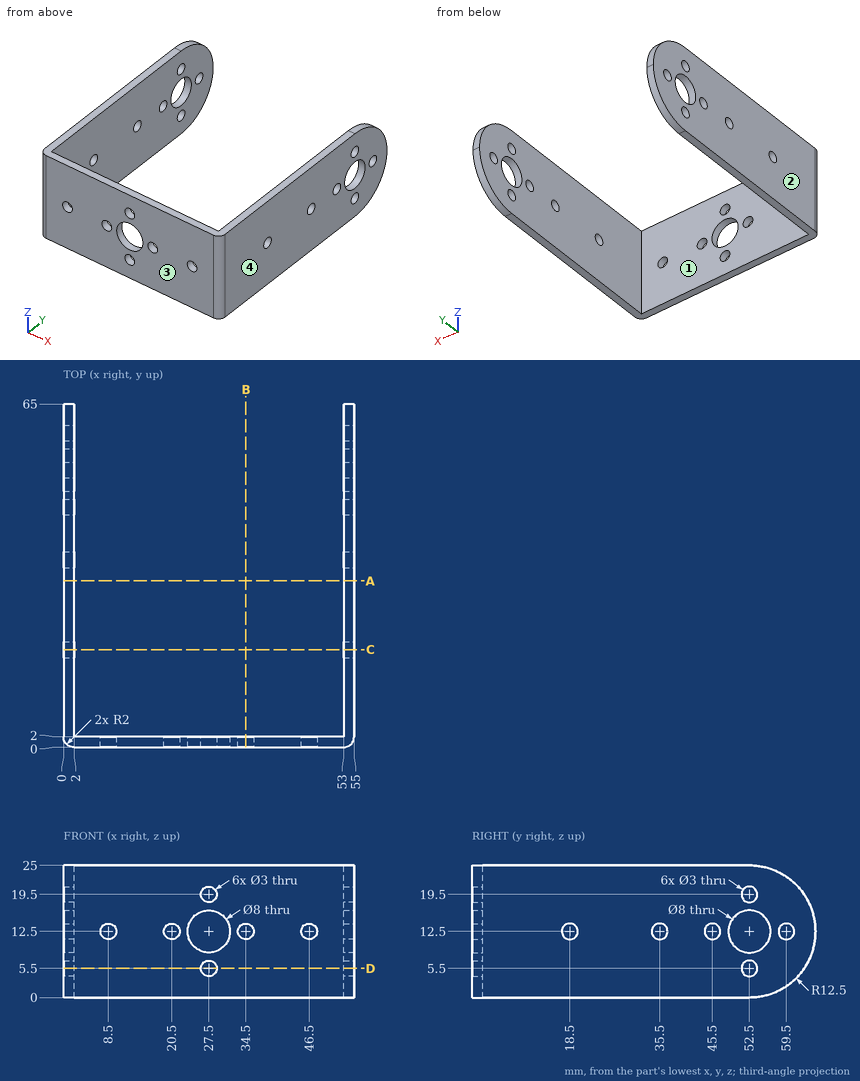
Could you check a few things on this drawing? It's one solid part, dimensions in mm from its lowest x, y, z. Give positions to 0.01 mm unless a question says otherwise; leave off trailing zeros. Write each loop counter-clockwise with the first axis right and the second up, starting at its lowest first coordinate (ties: lowest second). Pieces come first, ordered by that corner, then holes. Notation, with made-up numbers: (-26.75, 20) -> (1.25, 20) arc R13 ccw to (1.25, 37) -> close; hole circle Ø9 at (49, 37). An arc over 180 degrees is marked (long way). Write item = value, one per line.
(1) Suppose I cut it at B-B on x = 34.5. Write out the boundary of the cut face in (y, z).
Worked out:
outline = (0, 0) -> (2, 0) -> (2, 11) -> (0, 11) -> close; (0, 14) -> (2, 14) -> (2, 25) -> (0, 25) -> close
(2) I need wall thicknesses on probe 1 along Z at (x, y) = (27.5, 1.05); probe 2 along X at (y, z) = (59, 8); probe 3 along Y at (x, z) = (48, 6.25). Which ranges of each line are inside material? Lowest first, please. Write a range as from..to.
Worked out:
probe_1 = 0..4, 7..8.5, 16.5..18, 21..25
probe_2 = 0..2, 53..55
probe_3 = 0..2
(3) Thinking about a two-plate mould opening in X: for the marked faces 1, 2, 3 and 4, which applies, released by +X, released by -X, zero draft, split by the parting line, or undercut?
Worked out:
face_1 = undercut
face_2 = released by -X
face_3 = zero draft
face_4 = released by +X
(4) I'm going to push flat-ended pins straight in: P1, Ø2.5, axis at x = 20.5, z = 12.5, coming from the +Y side; P2, Ø6, axis at x = 34, z = 7.5, coming from the +Y side. Where does each tip first touch, or does it pass through?
Worked out:
P1 = through
P2 = 2
(5) Suppose I cut it at C-C on y = 18.5. Write out the boundary of the cut face in (x, z), then the cut area to 3 significant figures.
Worked out:
outline = (0, 0) -> (2, 0) -> (2, 11) -> (0, 11) -> close; (0, 14) -> (2, 14) -> (2, 25) -> (0, 25) -> close; (53, 0) -> (55, 0) -> (55, 11) -> (53, 11) -> close; (53, 14) -> (55, 14) -> (55, 25) -> (53, 25) -> close
area = 88.0 mm^2
(6) Suppose I cut it at A-A on y = 31.5. Write out the boundary of the cut face in (x, z), then the cut area to 3 significant figures.
Worked out:
outline = (0, 0) -> (2, 0) -> (2, 25) -> (0, 25) -> close; (53, 0) -> (55, 0) -> (55, 25) -> (53, 25) -> close
area = 100 mm^2
(7) Suppose I cut it at D-D on z = 5.5. Write out the boundary of the cut face in (x, y), then the cut area to 3 significant figures.
Worked out:
outline = (0, 2) arc R2 ccw to (2, 0) -> (26, 0) -> (26, 2) -> (2, 2) -> (2, 51) -> (0, 51) -> close; (0, 54) -> (2, 54) -> (2, 62.86) -> (0, 62.86) -> close; (29, 0) -> (53, 0) arc R2 ccw to (55, 2) -> (55, 51) -> (53, 51) -> (53, 2) -> (29, 2) -> close; (53, 54) -> (55, 54) -> (55, 62.86) -> (53, 62.86) -> close
area = 334 mm^2
